Design review of the part shown in the three views and the two pictorial views. Dimensions are in mm from the part's minimum x, y and z. Round coordinates to 2 decimals unless told otherwise and drop trailing zeros. Loops run counter-clockwise (first coordinate to the right, second up) from the corner with the lowest first, then second, coordinate; pieces in that order, holes last. Notation, with made-up numbers: M 86,-11.5 L 92,-11.5 A20 cw 92,8.5 Z; hole C 17,73 d7. An arc over 180 degrees is marked long. One line per question, with ' | ' between items.
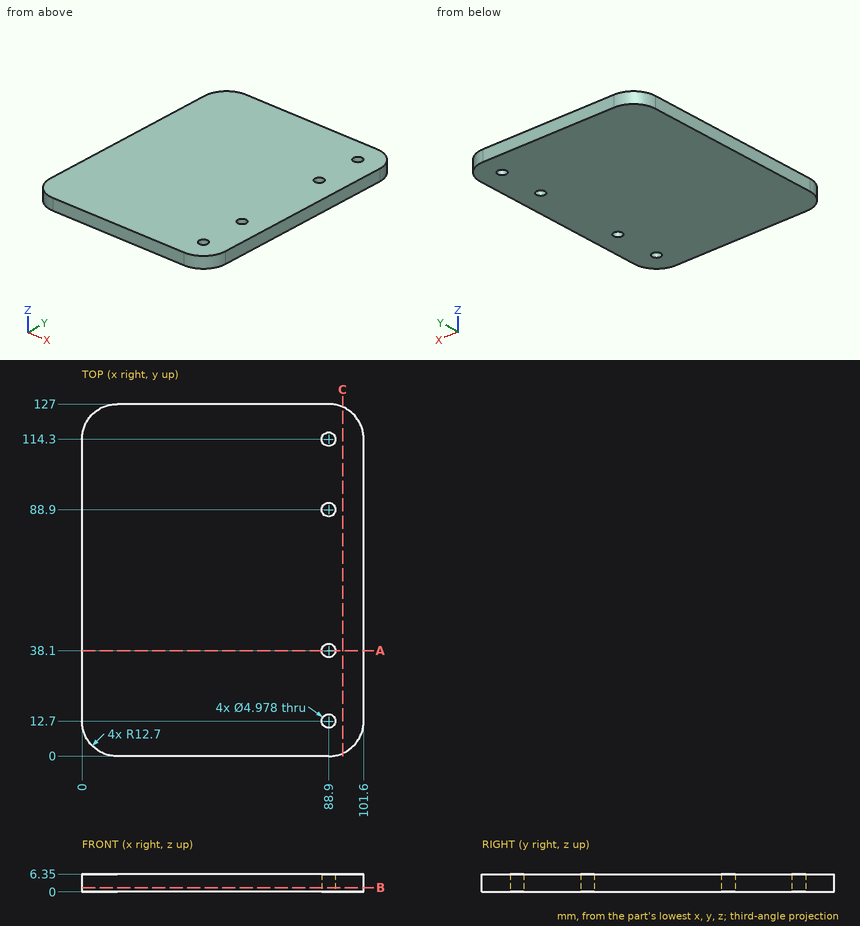
1) For line 1 (Y direction, x = 88.9, z = 4.5); line 2 (X direction, y = 91, z = 3.5) (1 decimal); line 3 (Y direction, x = 95, z = 4.75), list the stretches that pass through material, from the lowest coordinate up.
Output values:
line 1: y = 0 to 10.21, 15.19 to 35.61, 40.59 to 86.41, 91.39 to 111.81, 116.79 to 127 | line 2: x = 0 to 87.6, 90.2 to 101.6 | line 3: y = 1.56 to 125.44
2) Add section C-C on x = 94. State the section outline as (y, z) points.
Output values:
outline: M 1.07,0 L 125.93,0 L 125.93,6.35 L 1.07,6.35 Z
3) Add section B-B on z = 1.5. State the section outline as (x, y) points.
Output values:
outline: M 0,12.7 A12.7 ccw 12.7,0 L 88.9,0 A12.7 ccw 101.6,12.7 L 101.6,114.3 A12.7 ccw 88.9,127 L 12.7,127 A12.7 ccw 0,114.3 Z; hole C 88.9,12.7 d4.98; hole C 88.9,38.1 d4.98; hole C 88.9,88.9 d4.98; hole C 88.9,114.3 d4.98
4) Insertion check: P1, Ø5.5, axis at x = 88.9, y = 12.7, coming from the +Z side. The pin has a flat end and moves straight along its axis. Give the tip position at first contact, or say it passes through.
Output values:
P1: stops at z = 6.35
5) Add section A-A on y = 38.1. State the section outline as (x, z) points.
Output values:
outline: M 0,0 L 86.41,0 L 86.41,6.35 L 0,6.35 Z; M 91.39,0 L 101.6,0 L 101.6,6.35 L 91.39,6.35 Z
